Geometry check sheet. Reference: the model listing, model coordinates, mm. A direction names the side the tool comes from. Give positions to 0.01 mm unless a question says otherwise; leave off trailing zeros. Loops run counter-clockwise (first coordinate to the right, second up) from the corner with the lowest first, then second, coordinate; pieces in that order, holes last. Notation, with made-up numbers: (-13, 49) -> (21, 49) arc R28 ccw to (21, 69) -> close; hole circle Ø6 at (5, -2.75). An arc over 180 degrees is marked (long way). One line per item, written item: value. Start each with the question number.
(1) Sectioned sample at A-A, the plane y = -7. Record the cut outline in (x, z), then the cut area to 3 significant figures.
(2) Scan lines: line 1 along X through (y, z) = (3.75, -1.5); line 2 along Y through (x, z) = (-5, 2.5); line 3 along Y through (x, z) = (0, 1.25). Record each from-to range of solid material in increasing order. Write a range as from..to.
(3) Tool access check on faces 1 (the face through (0, -8.75, 0)), 2 (the face through (2.5, 1.25, -1.2)), 3 (the face through (2.25, 3.56, 0.01)). Record the directions out of +Z, -Z, +X, -X, +Y, -Y that give a thin tool (end or side, any length) a straight path to the whole face; none if there is none.
(4) Draft check along Z on faces 4 (the face through (0, 2.65, -5)), 5 (the face through (-0.75, 1.94, 5.7)), 6 (the face through (-0.01, 3.56, -1.75)). Enter one of: pulls with the +Z half, pulls with the -Z half, needs draft (parallel to the pull), parting line crosses it, or undercut.
(5) Gauge pin test, flat ends, axial feed: pin 1 Ø5 at (y, z) = (3, 4) entering from +X; pin 2 Ø2 at (x, z) = (-2, 3.5) entering from +Y; pin 3 Ø1 at (y, z) = (1.5, -3) entering from -X. Record the tip position at first contact, or that the pin passes through.
Autodesk Inventor part; units mm, degrees
ref_plane "Bolt_XY" through (0, 1.25, 0) normal (0, 1, 0) x (1, 0, 0)
ref_plane "Bolt_YZ" through (0, 1.25, 0) normal (1, 0, 0) x (0, 0, -1)
ref_plane "Bolt_ZX" through (0, 1.25, 0) normal (0, 0, -1) x (0, 1, 0)
sketch "Sketch_3" plane through (0, 0, 0) normal (0, 0, 1) x (1, 0, 0)
  line L0 (0, -8.75) -> (0, 4.45)
  line L1 (0, 4.45) -> (2.3483, 4.45)
  arc A0 (4.4749, 2.65) -> (2.3483, 4.45) centre (1.695, 1.522) ccw
  line L2 (4.4749, 2.65) -> (5.75, 2.65)
  line L3 (5.75, 2.65) -> (5.75, 1.25)
  line L4 (5.75, 1.25) -> (2.5, 1.25)
  line L5 (2.5, 1.25) -> (2.5, -8.2595)
  line L6 (2.5, -8.2595) -> (2.0095, -8.75)
  line L7 (2.0095, -8.75) -> (0, -8.75)
  line L8 (0, -8.75) -> (0, 4.45)
revolve "Revolution1" add sketch "Sketch_3" angle 360 about axis through (0, -8.75, 0) along (0, -1, 0)
thread "Thread1"
sketch "Sketch_1" plane through (0, 4.45, 0) normal (0, 1, 0) x (1, 0, 0)
  arc A0 (-1.9719, 0.4486) -> (-1.9719, -0.4486) centre (-1.7511, 0) ccw
  arc A1 (-1.3744, -1.4834) -> (-1.9719, -0.4486) centre (-2.4461, -1.4123) ccw
  arc A2 (-1.3744, -1.4834) -> (-0.5974, -1.932) centre (-0.8755, -1.5165) ccw
  arc A3 (0.5974, -1.932) -> (-0.5974, -1.932) centre (0, -2.8245) ccw
  arc A4 (0.5974, -1.932) -> (1.3744, -1.4834) centre (0.8755, -1.5165) ccw
  arc A5 (1.9719, -0.4486) -> (1.3744, -1.4834) centre (2.4461, -1.4123) ccw
  arc A6 (1.9719, -0.4486) -> (1.9719, 0.4486) centre (1.7511, 0) ccw
  arc A7 (1.3744, 1.4834) -> (1.9719, 0.4486) centre (2.4461, 1.4123) ccw
  arc A8 (1.3744, 1.4834) -> (0.5974, 1.932) centre (0.8755, 1.5165) ccw
  arc A9 (-0.5974, 1.932) -> (0.5974, 1.932) centre (0, 2.8245) ccw
  arc A10 (-0.5974, 1.932) -> (-1.3744, 1.4834) centre (-0.8755, 1.5165) ccw
  arc A11 (-1.9719, 0.4486) -> (-1.3744, 1.4834) centre (-2.4461, 1.4123) ccw
extrude "Extrusion1" cut sketch "Sketch_1" against normal blind 1.8
ref_plane "Bolt_XY" through (0, 1.25, 0) normal (0, 1, 0) x (1, 0, 0)
ref_plane "Bolt_YZ" through (0, 1.25, 0) normal (1, 0, 0) x (0, 0, -1)
ref_plane "Bolt_ZX" through (0, 1.25, 0) normal (0, 0, -1) x (0, 1, 0)
properties part number "0000-00082819_P2"
Calculated:
1. outline: circle Ø5 at (0, 0)
1. area: 19.6 mm2
2. line 1: x = -3.39..-1.38, 1.38..3.39
2. line 2: y = 1.25..2.65
2. line 3: y = -8.75..2.65
3. face 1: +Z, -Z, +X, -X, -Y
3. face 2: -Y
3. face 3: +Y
4. face 4: needs draft
4. face 5: parting line crosses it
4. face 6: undercut
5. pin 1: stops at x = 5.54
5. pin 2: stops at y = 4.21
5. pin 3: stops at x = -5.18
